from build123d import *

# Parameters (mm, degrees)
SKETCH_1_W          = 42
SKETCH_1_H          = 42
EXTRUDE_1_DEPTH     = 2
CHAMFER_1_SIZE      = 4
SKETCH_2_R          = 1.2
CUT_EXTRUDE_1_DEPTH = 2.5
SKETCH_3_R          = 15
CUT_EXTRUDE_2_DEPTH = 2.5
SKETCH_4_R          = 1.2
EXTRUDE_2_DEPTH     = 2
FILLET_1_R          = 4


with BuildPart() as part:
    # 草图1 → 凸台-拉伸1 (new body)
    with BuildSketch(Plane.XY):
        Rectangle(SKETCH_1_W, SKETCH_1_H)
    extrude(amount=EXTRUDE_1_DEPTH)

    # 倒角1
    chamfer_1_edges = [part.edges().sort_by_distance(p)[0] for p in [
        (21, -21, 1),
        (-21, -21, 1),
        (-21, 21, 1),
        (21, 21, 1),
    ]]
    chamfer(chamfer_1_edges, length=CHAMFER_1_SIZE)

    # 草图2 → 切除-拉伸1 (cut)
    with BuildSketch(Plane(origin=(0, 0, 0), x_dir=(-1, 0, 0), z_dir=(0, 0, -1))):
        with Locations((-15.55, 15.55)):
            Circle(SKETCH_2_R)
        with Locations((15.55, 15.55)):
            Circle(SKETCH_2_R)
        with Locations((15.55, -15.55)):
            Circle(SKETCH_2_R)
        with Locations((-15.55, -15.55)):
            Circle(SKETCH_2_R)
    extrude(amount=-CUT_EXTRUDE_1_DEPTH, mode=Mode.SUBTRACT)

    # 草图3 → 切除-拉伸2 (cut)
    with BuildSketch(Plane(origin=(0, 0, 0), x_dir=(-1, 0, 0), z_dir=(0, 0, -1))):
        Circle(SKETCH_3_R)
    extrude(amount=-CUT_EXTRUDE_2_DEPTH, mode=Mode.SUBTRACT)

    # 草图4 → 凸台-拉伸2 (add)
    with BuildSketch(Plane.XY):
        with BuildLine():
            Line((3.5, 23), (3.5, 19))
            Line((3.5, 19), (-3.5, 19))
            Line((-3.5, 19), (-3.5, 23))
            ThreePointArc((-3.5, 23), (0, 26.5), (3.5, 23))
        make_face()
        with Locations((0, 23)):
            Circle(SKETCH_4_R, mode=Mode.SUBTRACT)
        with BuildLine():
            ThreePointArc((3.5, -23), (0, -26.5), (-3.5, -23))
            Line((-3.5, -23), (-3.5, -19))
            Line((-3.5, -19), (3.5, -19))
            Line((3.5, -19), (3.5, -23))
        make_face()
        with Locations((0, -23)):
            Circle(SKETCH_4_R, mode=Mode.SUBTRACT)
        with BuildLine():
            ThreePointArc((-23, -3.5), (-26.5, 0), (-23, 3.5))
            Line((-23, 3.5), (-19, 3.5))
            Line((-19, 3.5), (-19, -3.5))
            Line((-19, -3.5), (-23, -3.5))
        make_face()
        with Locations((-23, 0)):
            Circle(SKETCH_4_R, mode=Mode.SUBTRACT)
        with BuildLine():
            Line((19, -3.5), (23, -3.5))
            ThreePointArc((23, -3.5), (26.5, 0), (23, 3.5))
            Line((23, 3.5), (19, 3.5))
            Line((19, 3.5), (19, -3.5))
        make_face()
        with Locations((23, 0)):
            Circle(SKETCH_4_R, mode=Mode.SUBTRACT)
    extrude(amount=EXTRUDE_2_DEPTH)

    # 圆角1
    fillet_1_edges = [part.edges().sort_by_distance(p)[0] for p in [
        (-21, 3.5, 1),
        (-21, -3.5, 1),
        (-3.5, -21, 1),
        (3.5, -21, 1),
        (21, -3.5, 1),
        (21, 3.5, 1),
        (3.5, 21, 1),
        (-3.5, 21, 1),
    ]]
    fillet(fillet_1_edges, radius=FILLET_1_R)


solid = part.part
The listing builds one solid part. Answer for the finished solid, in the listing's coordinates (mm). A direction names the side the tool comes from. Round coordinates to 2 decimals unless told otherwise and drop trailing zeros. Order: outer loops, then holes, each group sorted by start corner. A loop starts at its lowest first (then second) coordinate and runs counter-clockwise, first axis right, second up. Notation, with made-up numbers: M 79,6 L 108,6 A18 ccw 108,40 Z; hole C 77,85.25 d11. An arc over 180 degrees is marked long. Answer in a Markdown table with one row per item. Add a question column.
1) Flat-ended cylindrical pins translate along their axes: pin 1 Ø1 at (y, z) = (-13, 1.5) entering from -X; pin 2 Ø0.6 at (x, z) = (-12, 1) entering from -Y; pin 3 Ø1 at (y, z) = (-10, 1) entering from +X. Find the tip coordinate at first contact, or state that the pin passes through.
2) The part is cut by section A-A on x = 0. Determine the outline of the cut face in (y, z).
3) The part is cut by section C-C on z = 1.5. Count the separate pieces of the cut face and the enclosed holes in it, plus the area to 3 significant figures.
4) Consider line 1 along Y through (x, z) = (0, 1.4); line 2 along Y through (x, z) = (15.55, 0.5); line 3 along Y through (x, z) = (-1, 1.8). Determine where each line is inside the solid, lowest interval first. Write a range as from..to.
5) Determine the mould class of faces 1 (the face through (-21, -12, 1)), 2 (the face through (16.5, -16.28, 0.99)), 3 (the face through (12, -21, 1)) for opening direction Y: pulls with the +Y half, pulls with the -Y half, needs draft (parallel to the pull), parting line crosses it, or undercut.
6) The part is cut by section D-D on x = -18.5. Determine the outline of the cut face in (y, z).
7) The part is cut by section B-B on x = 12.5. Determine the outline of the cut face in (y, z).
8) Which of the six approach directions +Z, -Z, +X, -X, +Y, -Y give full straight-line access (tool end or side, diameter ignored) to faces 4 (the face through (21, 12, 1)), 5 (the face through (21, -12, 1)), 6 (the face through (-12, -21, 1)), 7 (the face through (-21, 12, 1))?
Findings below:
| question | item | result |
|---|---|---|
| 1 | pin 1 | stops at x = -21 |
| 1 | pin 2 | stops at y = -21 |
| 1 | pin 3 | stops at x = 21 |
| 2 | outline | M -26.5,0 L -24.2,0 L -24.2,2 L -26.5,2 Z; M -21.8,0 L -15,0 L -15,2 L -21.8,2 Z; M 15,0 L 21.8,0 L 21.8,2 L 15,2 Z; M 24.2,0 L 26.5,0 L 26.5,2 L 24.2,2 Z |
| 3 | separate pieces | 1 |
| 3 | enclosed holes | 9 |
| 3 | area | 1,140 mm² |
| 4 | line 1 | y = -26.5..-24.2, -21.8..-15, 15..21.8, 24.2..26.5 |
| 4 | line 2 | y = -21..-16.75, -14.35..14.35, 16.75..21 |
| 4 | line 3 | y = -26.35..-23.66, -22.34..-14.97, 14.97..22.34, 23.66..26.35 |
| 5 | face 1 | needs draft |
| 5 | face 2 | undercut |
| 5 | face 3 | pulls with the -Y half |
| 6 | outline | M -19.5,0 L 19.5,0 L 19.5,2 L -19.5,2 Z |
| 7 | outline | M -21,0 L -8.29,0 L -8.29,2 L -21,2 Z; M 8.29,0 L 21,0 L 21,2 L 8.29,2 Z |
| 8 | face 4 | +Z, -Z, +X, +Y |
| 8 | face 5 | +Z, -Z, +X, -Y |
| 8 | face 6 | +Z, -Z, -X, -Y |
| 8 | face 7 | +Z, -Z, -X, +Y |
